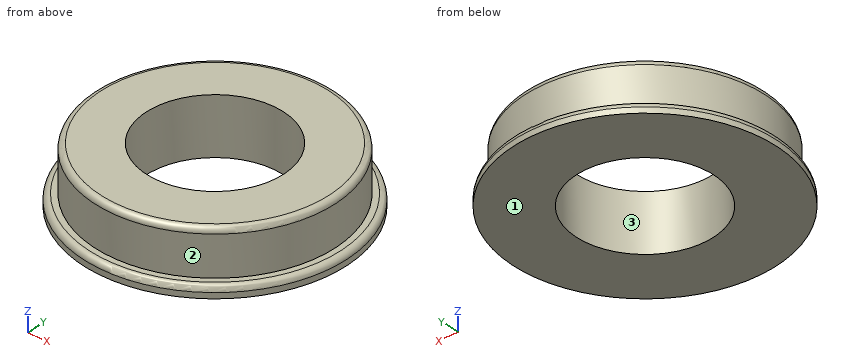
from build123d import *

# Parameters (mm, degrees)
SKETCH_1_R          = 11.5
EXTRUDE_1_DEPTH     = 1
SKETCH_2_R          = 10.5
EXTRUDE_2_DEPTH     = 4
SKETCH_3_R          = 6
CUT_EXTRUDE_1_DEPTH = 9
FILLET_1_R          = 0.5


with BuildPart() as part:
    # ｽｹｯﾁ1 → ﾎﾞｽ - 押し出し1 (new body)
    with BuildSketch(Plane.XY):
        Circle(SKETCH_1_R)
    extrude(amount=EXTRUDE_1_DEPTH)

    # ｽｹｯﾁ2 → ﾎﾞｽ - 押し出し2 (add)
    with BuildSketch(Plane.XY.offset(1)):
        Circle(SKETCH_2_R)
    extrude(amount=EXTRUDE_2_DEPTH)

    # ｽｹｯﾁ3 → ｶｯﾄ - 押し出し1 (cut)
    with BuildSketch(Plane.XY.offset(5)):
        Circle(SKETCH_3_R)
    extrude(amount=-CUT_EXTRUDE_1_DEPTH, mode=Mode.SUBTRACT)

    # ﾌｨﾚｯﾄ1
    fillet_1_edges = [part.edges().sort_by_distance(p)[0] for p in [
        (-11.5, 0, 1),
        (-10.5, 0, 5),
    ]]
    fillet(fillet_1_edges, radius=FILLET_1_R)


solid = part.part
Could you check a few things on this model? Use its own coordinates, in mm. Face numbers are marked on the shaded views. Give positions to 0.01 mm unless a question says otherwise; leave off trailing zeros. Loops run counter-clockwise (first coordinate to the right, second up) from the corner with the lowest first, then second, coordinate; pieces in that order, holes last. Notation, with made-up numbers: M -34,59.5 L -19,59.5 A29 cw -19,85.5 Z; hole C 39,87.25 d2. An arc over 180 degrees is marked long. Answer as a JSON object with one key per item and string values.
Q1. Suppose I cut it at A-A, the plane y = 0. List the corners of the cut face in (x, z) for me, plus the area to 3 significant figures.
Values found:
{"outline": "M -11.5,0 L -6,0 L -6,5 L -10,5 A0.5 ccw -10.5,4.5 L -10.5,1 L -11,1 A0.5 ccw -11.5,0.5 Z; M 6,0 L 11.5,0 L 11.5,0.5 A0.5 ccw 11,1 L 10.5,1 L 10.5,4.5 A0.5 ccw 10,5 L 6,5 Z", "area": "46.8 mm²"}
Q2. If we mould it in two halves opening along X, with no side actions, what happens to the marked faces 1, 2 and 3? For each: pulls with the +X half, pulls with the -X half, needs draft (parallel to the pull), parting line crosses it, or undercut.
Values found:
{"face 1": "needs draft", "face 2": "parting line crosses it", "face 3": "undercut"}
Q3. Suppose I cut it at C-C, the plane z = 2.7. List the corners of the cut face in (x, y) for me.
Values found:
{"outline": "C 0,0 d21; hole C 0,0 d12"}
Q4. For P1, Ø1, axis at y = 4, z = 4.5, coming from the +X side; P2, Ø3, axis at x = 6, z = 2, coming from the +Y side, each with a flat end and sliding along its axis, tell me the tip position at first contact or that it passes through.
Values found:
{"P1": "stops at x = 9.9", "P2": "stops at y = 10.2"}
Q5. If I drill on probe 1 along Y at (x, z) = (0, 2.1); probe 2 along Z at (x, y) = (-10.25, -3.5); probe 3 along Y at (x, z) = (4, 0.35), over which ranges is the centre line in solid material (lowest first)? Write a range as [from, to].
Values found:
{"probe 1": "y = [-10.5, -6], [6, 10.5]", "probe 2": "z = [0, 1]", "probe 3": "y = [-10.78, -4.47], [4.47, 10.78]"}
